Verification items for the finished model (mm, model axes). A direction names the side the tool comes from. Give positions to 0.01 mm unless a question says otherwise; leave off trailing zeros. Write each loop counter-clockwise with the first axis right and the second up, starting at its lowest first coordinate (ties: lowest second). Pieces come first, ordered by that corner, then holes. Notation, with made-up numbers: (-15.75, 1.5) -> (-4.75, 1.5) arc R18 ccw to (-4.75, 6.5) -> close; hole circle Ø8 at (63.25, 63.5). An arc over 180 degrees is marked (long way). Answer as CSV lines item,"result".
```python
from build123d import *

# Parameters (mm, degrees)
F0_R      = 1.1
F1_DEPTH  = 1.5
F3_DEPTH  = 1.5
F5_DEPTH  = 1.5
F6_R      = 1
F8_DEPTH  = 16.15
F11_R     = 1.1
F11_R_2   = 7.5
F12_DEPTH = 1.5


with BuildPart() as f1:
    # F0 (on Top) → F1 (new body)
    with BuildSketch(Plane.XY):
        with BuildLine():
            Line((16.5, 34.3955410847), (-16.5, 34.3955410847))
            Line((-16.5, 34.3955410847), (-16.5, -34.3955410847))
            Line((-16.5, -34.3955410847), (-10.5, -34.3955410847))
            Line((-10.5, -34.3955410847), (-10.5, -31.3955410847))
            ThreePointArc((-10.5, -31.3955410847), (-6.5, -27.3955410847), (-2.5, -31.3955410847))
            Line((-2.5, -31.3955410847), (-2.5, -34.3955410847))
            Line((-2.5, -34.3955410847), (16.5, -34.3955410847))
            Line((16.5, -34.3955410847), (16.5, 21.1730014102))
            Line((16.5, 21.1730014102), (13.5, 21.1730014102))
            ThreePointArc((13.5, 21.1730014102), (9.5, 25.1730014102), (13.5, 29.1730014102))
            Line((13.5, 29.1730014102), (16.5, 29.1730014102))
            Line((16.5, 29.1730014102), (16.5, 34.3955410847))
        make_face()
        with Locations((-12.7225396744, -31.3955410847)):
            Circle(F0_R, mode=Mode.SUBTRACT)
        with Locations((-10.9, -26.9955410847)):
            Circle(F0_R, mode=Mode.SUBTRACT)
        with Locations((-0.2774603256, -31.3955410847)):
            Circle(F0_R, mode=Mode.SUBTRACT)
        with Locations((-2.1, -26.9955410847)):
            Circle(F0_R, mode=Mode.SUBTRACT)
        with Locations((-6.5, -25.1730014102)):
            Circle(F0_R, mode=Mode.SUBTRACT)
        with Locations((7.2774603256, 25.1730014102)):
            Circle(F0_R, mode=Mode.SUBTRACT)
        with Locations((9.1, 20.7730014102)):
            Circle(F0_R, mode=Mode.SUBTRACT)
        with Locations((13.5, 18.9504617358)):
            Circle(F0_R, mode=Mode.SUBTRACT)
        with Locations((9.1, 29.5730014102)):
            Circle(F0_R, mode=Mode.SUBTRACT)
        with Locations((13.5, 31.3955410847)):
            Circle(F0_R, mode=Mode.SUBTRACT)
    extrude(amount=F1_DEPTH)

    # F2 (on face) → F3 (cut, through all)
    with BuildSketch(Plane.XY.offset(1.5)):
        Polygon((16.5, -34.3955410847), (16.5, 15.9504617358), (8.5, 3.9504617358), (2.7225396744, -34.3955410847), align=None)
        Polygon((-16.5, 9.3955410847), (-0.2225396744, 34.3955410847), (-16.5, 34.3955410847), align=None)
    extrude(amount=-F3_DEPTH, mode=Mode.SUBTRACT)

    # F4 (on face) → F5 (cut, through all)
    with BuildSketch(Plane.XY.offset(1.5)):
        with BuildLine():
            Line((-7.3635261338, 12.0333090433), (-0.2702674285, 22.9276048416))
            ThreePointArc((-0.2702674285, 22.9276048416), (-0.1298962002, 23.6799892884), (-0.5626548972, 24.3112628803))
            Line((-0.5626548972, 24.3112628803), (-0.7302594479, 24.4203899373))
            ThreePointArc((-0.7302594479, 24.4203899373), (-1.4826438948, 24.5607611656), (-2.1139174867, 24.1280024686))
            Line((-2.1139174867, 24.1280024686), (-9.2071761919, 13.2337066703))
            ThreePointArc((-9.2071761919, 13.2337066703), (-9.3475474202, 12.4813222235), (-8.9147887232, 11.8500486316))
            Line((-8.9147887232, 11.8500486316), (-8.7471841725, 11.7409215746))
            ThreePointArc((-8.7471841725, 11.7409215746), (-7.9947997256, 11.6005503463), (-7.3635261338, 12.0333090433))
        make_face()
        with BuildLine():
            ThreePointArc((2.8700363395, 18.5870607935), (2.1176518927, 18.7274320218), (1.4863783008, 18.2946733248))
            Line((1.4863783008, 18.2946733248), (-6.7901137686, 5.5830894784))
            ThreePointArc((-6.7901137686, 5.5830894784), (-7.3932540535, 4.2778380614), (-7.6, 2.8549130533))
            Line((-7.6, 2.8549130533), (-7.6, -19.1730014102))
            ThreePointArc((-7.6, -19.1730014102), (-7.3071067812, -19.8801081914), (-6.6, -20.1730014102))
            Line((-6.6, -20.1730014102), (-6.5, -20.1730014102))
            Line((-6.5, -20.1730014102), (-6.4, -20.1730014102))
            ThreePointArc((-6.4, -20.1730014102), (-5.6928932188, -19.8801081914), (-5.4, -19.1730014102))
            Line((-5.4, -19.1730014102), (-5.4, 2.2018212324))
            ThreePointArc((-5.4, 2.2018212324), (-5.1932540535, 3.6247462405), (-4.5901137686, 4.9299976575))
            Line((-4.5901137686, 4.9299976575), (3.330028359, 17.0942756977))
            ThreePointArc((3.330028359, 17.0942756977), (3.4703995873, 17.8466601446), (3.0376408903, 18.4779337365))
            Line((3.0376408903, 18.4779337365), (2.9538386149, 18.532497265))
            Line((2.9538386149, 18.532497265), (2.8700363395, 18.5870607935))
        make_face()
        with BuildLine():
            Line((-0.2, -2.1730014102), (-0.4, -2.1730014102))
            ThreePointArc((-0.4, -2.1730014102), (-1.1071067812, -2.4658946291), (-1.4, -3.1730014102))
            Line((-1.4, -3.1730014102), (-1.4, -16.1730014102))
            ThreePointArc((-1.4, -16.1730014102), (-1.1071067812, -16.8801081914), (-0.4, -17.1730014102))
            Line((-0.4, -17.1730014102), (-0.2, -17.1730014102))
            ThreePointArc((-0.2, -17.1730014102), (0.5071067812, -16.8801081914), (0.8, -16.1730014102))
            Line((0.8, -16.1730014102), (0.8, -3.1730014102))
            ThreePointArc((0.8, -3.1730014102), (0.5071067812, -2.4658946291), (-0.2, -2.1730014102))
        make_face()
    extrude(amount=-F5_DEPTH, mode=Mode.SUBTRACT)

    # F6
    f6_edges = [f1.edges().sort_by_distance(p)[0] for p in [
        (-16.5, -34.395541, 0.75),
        (-10.5, -34.395541, 0.75),
        (-2.5, -34.395541, 0.75),
        (2.72254, -34.395541, 0.75),
        (8.5, 3.950462, 0.75),
        (16.5, 15.950462, 0.75),
        (16.5, 34.395541, 0.75),
        (16.5, 21.173001, 0.75),
        (16.5, 29.173001, 0.75),
    ]]
    fillet(f6_edges, radius=F6_R)

    # F7 (on face) → F8 (join)
    with BuildSketch(Plane.XY.offset(1.5)):
        Polygon((-17.7570341306, 10.2139940122), (-16.5, 9.3955410847), (-0.2225396744, 34.3955410847), (-1.479573805, 35.2139940122), align=None)
    extrude(amount=-F8_DEPTH)

    # F10: F1 across plane


with BuildPart() as f1_1:
    add(f1.part)
    add(f1.part.mirror(Plane.XY.offset(-14.65)))

    # F11 (on face) → F12 (cut, through all)
    with BuildSketch(Plane(origin=(-17.1408454803, 11.1603772901, 0), x_dir=(-0.545635285, -0.8380227537, 0), z_dir=(-0.8380227537, 0.545635285, 0))):
        with Locations((-23.7867577831, -24.65)):
            Circle(F11_R)
        with Locations((-23.7867577831, -4.65)):
            Circle(F11_R)
        with Locations((-3.7867577831, -24.65)):
            Circle(F11_R)
        with Locations((-3.7867577831, -4.65)):
            Circle(F11_R)
        with Locations((-13.7867577831, -14.65)):
            Circle(F11_R_2)
    extrude(amount=-F12_DEPTH, mode=Mode.SUBTRACT)


solid = f1_1.part
```
1) Tool access check on faces 4 (the cylindrical face through (-6.588, -27.397, 0.74)), 5 (the flat face through (14, 29.173, 1)), 6 (the cylindrical face through (-8, 11.6, -30.1)). Record the directions out of +Z, -Z, +X, -X, +Y, -Y that give a thin tool (end or side, any length) a straight path to the whole face; none if there is none.
Reported:
face 4,"+Z, -Z, -Y"
face 5,"+Z, -Z, +X"
face 6,"+Z, -Z"
2) Section check C-C (z = -13). Record the boundary of the cut face in (x, y), and give its area (3 significant figures).
Reported:
outline,"(-17.76, 10.21) -> (-16.5, 9.4) -> (-12.35, 15.76) -> (-13.61, 16.58) -> close; (-5.63, 28.85) -> (-4.37, 28.03) -> (-0.22, 34.4) -> (-1.48, 35.21) -> close"
area,"22.8 mm²"
3) Section check B-B (y = 1.5). Record the boundary of the cut face in (x, z), and give its area (3 significant figures).
Reported:
outline,"(-16.5, -30.8) -> (-7.6, -30.8) -> (-7.6, -29.3) -> (-16.5, -29.3) -> close; (-16.5, 0) -> (-7.6, 0) -> (-7.6, 1.5) -> (-16.5, 1.5) -> close; (-5.4, -30.8) -> (8.13, -30.8) -> (8.13, -29.3) -> (-5.4, -29.3) -> close; (-5.4, 0) -> (8.13, 0) -> (8.13, 1.5) -> (-5.4, 1.5) -> close"
area,"67.3 mm²"
4) Section check A-A (z = -20). Record the boundary of the cut face in (x, y), and give its area (3 significant figures).
Reported:
outline,"(-17.76, 10.21) -> (-16.5, 9.4) -> (-11.23, 17.49) -> (-12.49, 18.31) -> close; (-6.75, 27.12) -> (-5.49, 26.3) -> (-0.22, 34.4) -> (-1.48, 35.21) -> close"
area,"29.0 mm²"
5) Scan lines: line 1 along Z through (x, y) = (7.5, 13.5); line 2 along Y through (x, z) = (-0.5, -22); line 3 along X through (y, z) = (11, -23). Record each from-to range of solid material in increasing order.
Reported:
line 1,"-30.8 to -29.3, 0 to 1.5"
line 2,"33.97 to 34.58"
line 3,"-17.25 to -15.46"
6) Section check D-D (z = -2). Record the boundary of the cut face in (x, y).
Reported:
outline,"(-17.76, 10.21) -> (-16.5, 9.4) -> (-0.22, 34.4) -> (-1.48, 35.21) -> close"
7) Depth check by flat-ended pin: pin 1 (1.6 mm diameter, centred on x = 14.5, z = 0.5, fed in from -Y); pin 2 (5 mm diameter, centred on y = 7.5, z = -7, fed in from +X); pin 3 (2 mm diameter, centred on y = 23.5, z = -24, fed in from -X). Enter the tip coordinate at first touch or a pass-through.
Reported:
pin 1,"y = 11.75"
pin 2,"x = -16.11"
pin 3,"x = -9.76"
8) Draft check along X on faces 1 (the flat face through (-5, 1, -30.8)), 2 (the cylindrical face through (9.5, 25.1, -30)), 3 (the cylindrical face through (8.86, 28.5, 0.74)). Enter one of: +X half, -X half, draft (parallel to the pull), parting line (faces both ways), or undercut.
Reported:
face 1,"draft"
face 2,"+X half"
face 3,"undercut"
